```python
from build123d import *

# Parameters (mm, degrees)
SKETCH1_W           = 6
SKETCH1_H           = 70
BOSS_EXTRUDE1_DEPTH = 5
SKETCH2_R           = 1.6
CUT_EXTRUDE1_DEPTH  = 36.482389998
SKETCH5_W           = 1.5
SKETCH5_H           = 40.4
BOSS_EXTRUDE2_DEPTH = 5
SKETCH7_W           = 14.889639403
SKETCH7_H           = 37
CUT_EXTRUDE5_DEPTH  = 3
SKETCH8_W           = 4
SKETCH8_H           = 21.6
CUT_EXTRUDE6_DEPTH  = 3
SKETCH9_W           = 16.5
SKETCH9_H           = 10
BOSS_EXTRUDE3_DEPTH = 6
SKETCH6_R           = 1.3
CUT_EXTRUDE4_DEPTH  = 40.092838219
SKETCH10_R          = 1.6
CUT_EXTRUDE7_DEPTH  = 9
CUT_EXTRUDE8_DEPTH  = 3.5
BOSS_EXTRUDE4_DEPTH = 6
CUT_EXTRUDE10_REACH = 41.093
BOSS_EXTRUDE5_DEPTH = 10.5
FILLET3_R           = 0.75
SKETCH16_W          = 7.5
SKETCH16_H          = 2.1
BOSS_EXTRUDE6_DEPTH = 2


with BuildPart() as part:
    # Sketch1 → Boss-Extrude1 (new body)
    with BuildSketch(Plane(origin=(0, 0, 0), x_dir=(1, 0, 0), z_dir=(0, 1, 0))):
        Rectangle(SKETCH1_W, SKETCH1_H)
    extrude(amount=BOSS_EXTRUDE1_DEPTH)

    # Sketch2 → Cut-Extrude1 (cut, through all)
    with BuildSketch(Plane(origin=(0, 5, 0), x_dir=(1, 0, 0), z_dir=(0, 1, 0))):
        with Locations(Location((0, -32, 0), (0, 0, 270))):
            Circle(SKETCH2_R)
        with Locations(Location((0, 32, 0), (0, 0, 270))):
            Circle(SKETCH2_R)
    extrude(amount=-CUT_EXTRUDE1_DEPTH, mode=Mode.SUBTRACT)

    # Sketch5 → Boss-Extrude2 (add)
    with BuildSketch(Plane(origin=(0, 5, 0), x_dir=(1, 0, 0), z_dir=(0, 1, 0))):
        with Locations((-3.75, 0)):
            Rectangle(SKETCH5_W, SKETCH5_H)
    extrude(amount=-BOSS_EXTRUDE2_DEPTH)

    # Sketch7 → Cut-Extrude5 (cut)
    with BuildSketch(Plane(origin=(0, 5, 0), x_dir=(1, 0, 0), z_dir=(0, 1, 0))):
        with Locations((-6.444819702, 0)):
            Rectangle(SKETCH7_W, SKETCH7_H)
    extrude(amount=-CUT_EXTRUDE5_DEPTH, mode=Mode.SUBTRACT)

    # Sketch8 → Cut-Extrude6 (cut)
    with BuildSketch(Plane(origin=(0, 2, 0), x_dir=(1, 0, 0), z_dir=(0, 1, 0))):
        with Locations((-2.5, 0)):
            Rectangle(SKETCH8_W, SKETCH8_H)
    extrude(amount=-CUT_EXTRUDE6_DEPTH, mode=Mode.SUBTRACT)

    # Sketch9 → Boss-Extrude3 (add)
    with BuildSketch(Plane.XZ):
        with Locations((-5.25, -18.5)):
            Rectangle(SKETCH9_W, SKETCH9_H)
    extrude(amount=BOSS_EXTRUDE3_DEPTH)

    # Sketch6 → Cut-Extrude4 (cut, through all)
    with BuildSketch(Plane(origin=(0, 5, 0), x_dir=(1, 0, 0), z_dir=(0, 1, 0))):
        with Locations(Location((-2, 15.5, 0), (0, 0, 90))):
            Circle(SKETCH6_R)
        with Locations(Location((-2, -15.5, 0), (0, 0, 270))):
            Circle(SKETCH6_R)
    extrude(amount=-CUT_EXTRUDE4_DEPTH, mode=Mode.SUBTRACT)

    # Sketch10 → Cut-Extrude7 (cut)
    with BuildSketch(Plane(origin=(0, 0, 0), x_dir=(1, 0, 0), z_dir=(0, 1, 0))):
        with Locations(Location((-11, 18, 0), (0, 0, 270))):
            Circle(SKETCH10_R)
    extrude(amount=-CUT_EXTRUDE7_DEPTH, mode=Mode.SUBTRACT)

    # Sketch11 → Cut-Extrude8 (cut)
    with BuildSketch(Plane(origin=(0, 0, 0), x_dir=(1, 0, 0), z_dir=(0, 1, 0))):
        Polygon((-13.5, 13.5), (-4.5, 13.5), (-4.5, 20.2), (-3, 20.2), (-3, 23.5), (-13.5, 23.5), align=None)
    extrude(amount=-CUT_EXTRUDE8_DEPTH, mode=Mode.SUBTRACT)

    # Sketch13 → Boss-Extrude4 (add)
    with BuildSketch(Plane(origin=(3, 0, 0), x_dir=(0, 0, -1), z_dir=(1, 0, 0))):
        Polygon((23.5, -6), (29.5, 0), (23.5, 0), align=None)
    extrude(amount=-BOSS_EXTRUDE4_DEPTH)

    # Cut-Extrude10: up to this face of the body (flat: up to its plane)
    cut_extrude10_end = Plane(part.part.faces().sort_by_distance((0.153252085, 0, 12.233088701))[0])
    # Sketch14 → Cut-Extrude10 (cut, up to the picked face)
    with BuildSketch(Plane.XZ.offset(6), mode=Mode.PRIVATE) as cut_extrude10_sk1:
        Polygon((-4.5, -18.1), (5.195583007, -18.1), (5.195583007, -13.5), (-9.1, -13.5), align=None)
    cut_extrude10_tool1 = split(extrude(cut_extrude10_sk1.sketch, amount=-CUT_EXTRUDE10_REACH, mode=Mode.PRIVATE), bisect_by=cut_extrude10_end, keep=Keep.BOTH, mode=Mode.PRIVATE)
    add(cut_extrude10_tool1.solids().sort_by(Axis((-0.875708, -6, -15.653001), (0, 1, 0)))[0], mode=Mode.SUBTRACT)

    # Sketch15 → Boss-Extrude5 (add)
    with BuildSketch(Plane.ZY.offset(3)):
        Polygon((-23.5, -3.5), (-23.5, -6), (-26, -3.5), align=None)
    extrude(amount=BOSS_EXTRUDE5_DEPTH)

    # Fillet3
    fillet3_edges = [part.edges().sort_by_distance(p)[0] for p in [
        (-13.5, -4.75, -13.5),
    ]]
    fillet(fillet3_edges, radius=FILLET3_R)

    # Sketch16 → Boss-Extrude6 (add)
    with BuildSketch(Plane.XZ):
        with Locations((-0.75, -19.15)):
            Rectangle(SKETCH16_W, SKETCH16_H)
        with Locations((-0.75, -11.85)):
            Rectangle(SKETCH16_W, SKETCH16_H)
        with Locations((-0.75, 11.85)):
            Rectangle(SKETCH16_W, SKETCH16_H)
        with Locations((-0.75, 19.15)):
            Rectangle(SKETCH16_W, SKETCH16_H)
    extrude(amount=BOSS_EXTRUDE6_DEPTH)


solid = part.part
```
CAD build for the part. Positions are in the model's coordinates, mm. A direction names the side the tool comes from. Give positions to 0.01 mm unless a question says otherwise; leave off trailing zeros. Loops run counter-clockwise (first coordinate to the right, second up) from the corner with the lowest first, then second, coordinate; pieces in that order, holes last. Notation, with made-up numbers: (-13, 44) - (15, 44) arc R24 cw to (15, 66) - close; hole circle Ø11 at (74.25, 35.25). An arc over 180 degrees is marked (long way). Put each result on its own line as item: value.
Q1. Slice it at D-D (x = -11). Give the cut face in (y, z), plus the area to 3 significant figures.
Filled in:
outline: (-6, -23.5) - (-3.5, -26) - (-3.5, -19.6) - (-6, -19.6) - close; (-6, -16.4) - (-3.5, -16.4) - (-3.5, -13.5) - (-6, -13.5) - close
area: 20.1 mm²
Q2. Slice it at B-B (z = -32). Give the cut face in (x, y), plus the area to 3 significant figures.
Filled in:
outline: (-3, 0) - (-1.6, 0) - (-1.6, 5) - (-3, 5) - close; (1.6, 0) - (3, 0) - (3, 5) - (1.6, 5) - close
area: 14.0 mm²
Q3. Flat gauge pins, fed straight in: pin 1 (1 mm diameter, centred on x = -1.5, y = -1, fed in from -Z); pin 2 (2.5 mm diameter, centred on x = -1, z = -16.5, fed in from -Y); pin 3 (5.5 mm diameter, centred on y = 2, z = 13.5, fed in from -X). Where does each tip first touch, or does it go through?
Filled in:
pin 1: stops at z = -29
pin 2: stops at y = 0
pin 3: stops at x = -4.5
Q4. Mould opens along X. For faces 4 (the face through (-0.5, 1, 0)), 5 (the face through (0.07, 2.54, -33.6)), 6 (the face through (-2, 0, -10.8)) say: pulls with the +X half, pulls with the -X half, needs draft (parallel to the pull), parting line crosses it, or undercut.
Filled in:
face 4: pulls with the -X half
face 5: undercut
face 6: needs draft
Q5. Slice it at A-A (y = -1.25). Give the cut face in (x, z), plus the area to 3 significant figures.
Filled in:
outline: (-4.5, -20.2) - (-3, -20.2) - (-3, -28.25) - (3, -28.25) - (3, -18.1) - (-4.5, -18.1) - close; (-4.5, -12.9) - (3, -12.9) - (3, -10.8) - (-4.5, -10.8) - close; (-4.5, 10.8) - (3, 10.8) - (3, 12.9) - (-4.5, 12.9) - close; (-4.5, 18.1) - (3, 18.1) - (3, 20.2) - (-4.5, 20.2) - close
area: 111 mm²
Q6. Tool access for faces 1 (the face through (-1, -3, -18.1)), 2 (the face through (-2, 4, 18.5)), 3 (the face through (-1, -2, -12)): list every direction of +Z, -Z, +X, -X, +Y, -Y with a clear straight run to the whole face (end or side of a thin tool).
Filled in:
face 1: +X, -Y
face 2: -X, +Y
face 3: +Z, +X, -X, -Y
Q7. Probe line 1 along X through (y, z) = (1.5, -15.5); line 2 along Y through (x, z) = (-11, -25); line 3 along Y through (x, z) = (1.5, -29.5). List the from-to ranges inside material, lowest first.
Filled in:
line 1: x = -4.5 to -3.3, -0.7 to 3
line 2: y = -4.5 to -3.5
line 3: y = 0 to 5
Q8. Slice it at C-C (z = -15.5). Give the cut face in (x, y), plus the area to 3 significant figures.
Filled in:
outline: (-13.5, -6) - (-7.1, -6) - (-7.1, -3.5) - (-13.5, -3.5) - close; (-4.5, 0) - (-3.3, 0) - (-3.3, 2) - (-4.5, 2) - close; (-0.7, 0) - (3, 0) - (3, 5) - (1, 5) - (1, 2) - (-0.7, 2) - close
area: 31.8 mm²
